Can you work these out from the model? Positions are in its coordinate system, mm. A direction names the side the tool comes from. Give positions to 0.01 mm unless a question says otherwise; leave off trailing zeros. Order: outer loops, then holes, each group sorted by start corner. A loop starts at its lowest first (then second) coordinate and runs counter-clockwise, first axis right, second up. Notation, with made-up numbers: (32.25, 6.25) - (53.25, 6.25) arc R12 ccw to (53.25, 12.25) - close; hole circle Ø5 at (-23, -33). An arc over 180 degrees is marked (long way). Return JSON: item names as keys, results as strings.
```python
from build123d import *

# Parameters (mm, degrees)
F1_DEPTH = 25
F2_DEPTH = 8
F3_W     = 13.941449
F3_H     = 11.943896
F4_DEPTH = 25


with BuildPart() as f1:
    # F0 (on Front) → F1 (new body)
    with BuildSketch(Plane.XZ):
        with BuildLine():
            Line((-31.05, 4), (-31.05, 0))
            Line((-31.05, 0), (31.05, 0))
            Line((31.05, 0), (31.05, 4))
            Line((31.05, 4), (27.55, 4))
            Line((27.55, 4), (27.55, 6.9))
            Line((27.55, 6.9), (0, 6.9))
            Line((0, 6.9), (0, 27.01417))
            Line((0, 27.01417), (-27.55, 27.01417))
            Line((-27.55, 27.01417), (-27.55, 9.67))
            Line((-27.55, 9.67), (-18.593099, 9.67))
            ThreePointArc((-18.593099, 9.67), (-18.210415, 9.74612), (-17.885992, 9.962893))
            Line((-17.885992, 9.962893), (-11.474443, 16.374443))
            ThreePointArc((-11.474443, 16.374443), (-2.422469, 14.573893), (-7.55, 6.9))
            Line((-7.55, 6.9), (-27.55, 6.9))
            Line((-27.55, 6.9), (-27.55, 4))
            Line((-27.55, 4), (-31.05, 4))
        make_face()
        with BuildLine():
            Line((-27.55, 9.67), (-27.55, 6.9))
            Line((-27.55, 6.9), (-7.55, 6.9))
            ThreePointArc((-7.55, 6.9), (-2.422469, 14.573893), (-11.474443, 16.374443))
            Line((-11.474443, 16.374443), (-17.885992, 9.962893))
            ThreePointArc((-17.885992, 9.962893), (-18.210415, 9.74612), (-18.593099, 9.67))
            Line((-18.593099, 9.67), (-27.55, 9.67))
        make_face()
        with BuildLine():
            Line((-7.55, 8.7), (-14.189087, 8.7))
            ThreePointArc((-14.189087, 8.7), (-15.112967, 9.317317), (-14.896194, 10.407107))
            Line((-14.896194, 10.407107), (-10.20165, 15.10165))
            ThreePointArc((-10.20165, 15.10165), (-4.085452, 13.885063), (-7.55, 8.7))
        make_face(mode=Mode.SUBTRACT)
        with BuildLine():
            ThreePointArc((-14.896194, 10.407107), (-15.112967, 9.317317), (-14.189087, 8.7))
            Line((-14.189087, 8.7), (-7.55, 8.7))
            ThreePointArc((-7.55, 8.7), (-4.085452, 13.885063), (-10.20165, 15.10165))
            Line((-10.20165, 15.10165), (-14.896194, 10.407107))
        make_face()
    extrude(amount=F1_DEPTH)

    # F0 (on Front) → F2 (cut)
    with BuildSketch(Plane.XZ):
        with BuildLine():
            Line((-27.55, 9.67), (-27.55, 6.9))
            Line((-27.55, 6.9), (-7.55, 6.9))
            ThreePointArc((-7.55, 6.9), (-2.422469, 14.573893), (-11.474443, 16.374443))
            Line((-11.474443, 16.374443), (-17.885992, 9.962893))
            ThreePointArc((-17.885992, 9.962893), (-18.210415, 9.74612), (-18.593099, 9.67))
            Line((-18.593099, 9.67), (-27.55, 9.67))
        make_face()
        with BuildLine():
            Line((-7.55, 8.7), (-14.189087, 8.7))
            ThreePointArc((-14.189087, 8.7), (-15.112967, 9.317317), (-14.896194, 10.407107))
            Line((-14.896194, 10.407107), (-10.20165, 15.10165))
            ThreePointArc((-10.20165, 15.10165), (-4.085452, 13.885063), (-7.55, 8.7))
        make_face(mode=Mode.SUBTRACT)
    extrude(amount=F2_DEPTH, mode=Mode.SUBTRACT)

    # F3 (on face) → F4 (join)
    with BuildSketch(Plane.YZ):
        with Locations((-12.311068, 16.862532)):
            Rectangle(F3_W, F3_H)
    extrude(amount=F4_DEPTH)


solid = f1.part
```
1. Suppose I cut it at D-D (x = -24). List the corners of the cut face in (y, z) for me.
Checks:
{"outline": "(-25, 0) - (0, 0) - (0, 6.9) - (-8, 6.9) - (-8, 9.67) - (0, 9.67) - (0, 27.01) - (-25, 27.01) - close"}
2. If I drill on L1, parallel to X at y = -4, z = 12.45; L2, parallel to X at y = -5.75, z = 12.45; L3, parallel to Y at x = 0.5, z = 18.5, over which ranges is the centre line in solid material (lowest first)? Write a range as [from, to].
Checks:
{"L1": "[-27.55, -15.4], [-12.85, -3.8], [-2, 0]", "L2": "[-27.55, -15.4], [-12.85, -3.8], [-2, 25]", "L3": "[-19.28, -5.34]"}
3. Suppose I cut it at C-C (y = -12.25). List the corners of the cut face in (x, z) for me.
Checks:
{"outline": "(-31.05, 0) - (31.05, 0) - (31.05, 4) - (27.55, 4) - (27.55, 6.9) - (0, 6.9) - (0, 10.89) - (25, 10.89) - (25, 22.83) - (0, 22.83) - (0, 27.01) - (-27.55, 27.01) - (-27.55, 4) - (-31.05, 4) - close"}
4. Suppose I cut it at A-A (x = 13). List the corners of the cut face in (y, z) for me.
Checks:
{"outline": "(-25, 0) - (0, 0) - (0, 6.9) - (-25, 6.9) - close; (-19.28, 10.89) - (-5.34, 10.89) - (-5.34, 22.83) - (-19.28, 22.83) - close"}
5. Suppose I cut it at B-B (y = -6.75). List the corners of the cut face in (x, z) for me.
Checks:
{"outline": "(-31.05, 0) - (31.05, 0) - (31.05, 4) - (27.55, 4) - (27.55, 6.9) - (0, 6.9) - (0, 10.89) - (25, 10.89) - (25, 22.83) - (0, 22.83) - (0, 27.01) - (-27.55, 27.01) - (-27.55, 9.67) - (-18.59, 9.67) arc R1 ccw to (-17.89, 9.96) - (-11.47, 16.37) arc R5.55 cw (long way) to (-7.55, 6.9) - (-27.55, 6.9) - (-27.55, 4) - (-31.05, 4) - close; (-14.9, 10.41) arc R1 ccw to (-14.19, 8.7) - (-7.55, 8.7) arc R3.75 ccw (long way) to (-10.2, 15.1) - close"}
6. For pin 1 Ø4 at (y, z) = (-3, 17.5) entering from +X; pin 2 Ø6 at (x, z) = (13, 17.5) entering from +Y; pin 3 Ø7 at (x, y) = (14.5, -12.5) entering from +Z, each with a flat end and sliding along its axis, tell me the tip position at first contact or that it passes through.
Checks:
{"pin 1": "x = 0", "pin 2": "y = -5.34", "pin 3": "z = 22.83"}
7. On a 3-axis mill with a long thin cutter (end or side, diameter ignored), from which of +Z, -Z, +X, -X, +Y, -Y can I reach the whole of each face in a straight line? I mean faces 4 (the face through (-27.55, -12, 16)), 5 (the face through (25, -12, 17)), 6 (the face through (-18, -4, 6.9)), 7 (the face through (12, -5.34, 17)), 8 (the face through (-4.126, -3.944, 13.98)). Say none if no direction works.
Checks:
{"face 4": "+Z, -X, +Y, -Y", "face 5": "+Z, +X, +Y, -Y", "face 6": "-X, +Y", "face 7": "+Z, +X, +Y", "face 8": "+Y"}
8. Thinking about a two-plate mould opening in Z: for faces 1 (the face through (-14, -12, 27.014)), 2 (the face through (-14.64, -3.94, 13.21)), 3 (the face through (31.05, -12, 2)), which applies, +Z half, -Z half, draft (parallel to the pull), parting line (faces both ways), or undercut?
Checks:
{"face 1": "+Z half", "face 2": "undercut", "face 3": "draft"}
